```python
from build123d import *

# Parameters (mm, degrees)
PAD_DEPTH       = 37.75
SKETCH001_R     = 0.75
SKETCH001_W     = 16.9
SKETCH001_H     = 5.75
SKETCH001_W_2   = 15.65
SKETCH001_H_2   = 6.05
POCKET_DEPTH    = 5
SKETCH003_R     = 2.4
SKETCH003_W     = 24
SKETCH003_H     = 7.75
PAD001_DEPTH    = 4.95
POCKET001_DEPTH = 4.9
SKETCH004_W     = 0.9
SKETCH004_H     = 10.5
PAD002_DEPTH    = 4.62


with BuildPart() as part:
    # Sketch → Pad (new body)
    with BuildSketch(Plane.XY):
        Polygon((-31, 20), (90, 20), (90, 19.1), (-30.1, 19.1), (-30.1, 7.3), (-31, 7.3), align=None)
    extrude(amount=PAD_DEPTH)

    # Sketch001 (on Face3 of Pad) → Pocket (cut)
    with BuildSketch(Plane.XZ.offset(-19.1)):
        with Locations((71.17, 37.5)):
            Circle(SKETCH001_R)
        Polygon((90, 34.175), (90, 24.025), (83, 24.025), (78.8, 19.825), (78.8, 17.925), (83, 13.725), (90, 13.725), (90, 3.575), (82.75, 3.575), (79.175, 0), (79.175, -11.454838), (99.765602, -11.454838), (99.765602, 41.466698), (78.897491, 41.466698), (79.175, 37.75), (82.75, 34.175), align=None)
        with Locations((14.05, 6.225)):
            Rectangle(SKETCH001_W, SKETCH001_H)
        with Locations((-15.375, 6.075)):
            Rectangle(SKETCH001_W_2, SKETCH001_H_2)
    extrude(amount=-POCKET_DEPTH, mode=Mode.SUBTRACT)

    # Sketch003 → Pad001 (join)
    with BuildSketch(Plane.XZ.offset(-19.1)):
        with Locations((67.8, 7.925)):
            Circle(SKETCH003_R)
        with Locations((35.6, 7.925)):
            Circle(SKETCH003_R)
        with Locations((51.7, 7.925)):
            Rectangle(SKETCH003_W, SKETCH003_H)
    extrude(amount=PAD001_DEPTH)

    # Sketch001 (on Face3 of Pad) → Pocket001 (cut)
    with BuildSketch(Plane.XZ.offset(-19.1)):
        with Locations((71.17, 37.5)):
            Circle(SKETCH001_R)
        Polygon((90, 34.175), (90, 24.025), (83, 24.025), (78.8, 19.825), (78.8, 17.925), (83, 13.725), (90, 13.725), (90, 3.575), (82.75, 3.575), (79.175, 0), (79.175, -11.454838), (99.765602, -11.454838), (99.765602, 41.466698), (78.897491, 41.466698), (79.175, 37.75), (82.75, 34.175), align=None)
        with Locations((14.05, 6.225)):
            Rectangle(SKETCH001_W, SKETCH001_H)
        with Locations((-15.375, 6.075)):
            Rectangle(SKETCH001_W_2, SKETCH001_H_2)
    extrude(amount=-POCKET001_DEPTH, mode=Mode.SUBTRACT)

    # Sketch004 (on Face2 of Pocket001) → Pad002 (join)
    with BuildSketch(Plane(origin=(0, 0, 0), x_dir=(1, 0, 0), z_dir=(0, 0, -1))):
        with Locations((-30.55, -12.55)):
            Rectangle(SKETCH004_W, SKETCH004_H)
    extrude(amount=PAD002_DEPTH)


solid = part.part
```
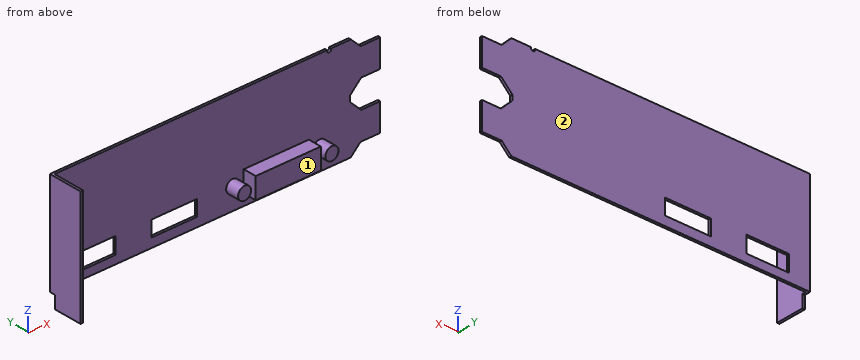
CAD build for the part. Positions are in the model's coordinates, mm. Face numbers are marked on the shaded views. A direction names the side the tool comes from. Round coordinates to 2 decimals unless told otherwise and drop trailing zeros. Write each loop counter-clockwise with the first axis right and the second up, starting at its lowest first coordinate (ties: lowest second). Pieces come first, ordered by that corner, then holes. Notation, with made-up numbers: (5, 71.25) -> (33, 71.25) arc R10 cw to (33, 77.25) -> close; hole circle Ø11 at (-23.5, 57.25). An arc over 180 degrees is marked (long way). Answer in a Markdown table with one row per item. Add a question column.
Item 1: Saw through at C-C, the plane y = 11.75. Write the cut outline in (x, z).
Item 2: Which spindle directions (+Z, -Z, +X, -X, +Y, -Y) get a long thin tool onto all of the face, cutting with end or side? Do the marked faces 1 and 2. Say none if no direction does.
Item 3: Saw through at D-D, the plane x = 35.6. Write the cut outline in (y, z) (3 decimals).
Item 4: Saw through at B-B, the plane x = 49. Write the cut outline in (y, z).
Item 5: Drill centre lines: line 1 (X direction, y = 17.25, z = 8); line 2 (X direction, y = 11, z = 25); line 3 (Y direction, x = 68, z = 34). Where is each one in solid material? Low to high. Write a range as from..to.
Item 6: Drop flat-ended pins along their axis: pin 1 Ø4 at (y, z) = (16.5, 7.5) entering from +X; pin 2 Ø11.5 at (x, z) = (34.5, 10.5) entering from -Y; pin 3 Ø0.7 at (x, y) = (12, 19.5) entering from -Z. Give the stop position or say it passes through.
Item 7: Saw through at A-A, the plane x = -11. Write the cut outline in (y, z), then the cut area to 3 significant figures.
Findings below:
| question | item | result |
|---|---|---|
| 1 | outline | (-31, -4.62) -> (-30.1, -4.62) -> (-30.1, 37.75) -> (-31, 37.75) -> close |
| 2 | face 1 | +Z, -Z, +X, -Y |
| 2 | face 2 | +Z, -Z, +X, -X, +Y |
| 3 | outline | (14.15, 5.525) -> (19.1, 5.525) -> (19.1, 0) -> (20, 0) -> (20, 37.75) -> (19.1, 37.75) -> (19.1, 10.325) -> (14.15, 10.325) -> close |
| 4 | outline | (14.15, 4.05) -> (19.1, 4.05) -> (19.1, 0) -> (20, 0) -> (20, 37.75) -> (19.1, 37.75) -> (19.1, 11.8) -> (14.15, 11.8) -> close |
| 5 | line 1 | x = -31..-30.1, 33.2..38, 39.7..63.7, 65.4..70.2 |
| 5 | line 2 | x = -31..-30.1 |
| 5 | line 3 | y = 19.1..20 |
| 6 | pin 1 | stops at x = 70.2 |
| 6 | pin 2 | stops at y = 14.15 |
| 6 | pin 3 | stops at z = 0 |
| 7 | outline | (19.1, 0) -> (20, 0) -> (20, 3.05) -> (19.1, 3.05) -> close; (19.1, 9.1) -> (20, 9.1) -> (20, 37.75) -> (19.1, 37.75) -> close |
| 7 | area | 28.5 mm^2 |
